```python
from build123d import *

# Parameters (mm, degrees)
EXTRUDE_1_DEPTH          = 2.5
SKETCH_4_R               = 1.6
CUT_EXTRUDE_1_DEPTH      = 2.5
SKETCH_6_R               = 29
SKETCH_6_R_2             = 27.5
EXTRUDE_2_DEPTH          = 20
CUT_EXTRUDE_2_DEPTH      = 86.473878076
CUT_EXTRUDE_2_DEPTH_BACK = 86.473878076
SKETCH_7_W               = 18
SKETCH_7_H               = 8


with BuildPart() as part:
    # 草图2 → 凸台-拉伸1 (new body)
    with BuildSketch(Plane(origin=(0, 0, 0), x_dir=(1, 0, 0), z_dir=(0, 1, 0))):
        Polygon((-42.5, 21.336828309), (42.5, 21.336828309), (42.5, -70.663171691), (32.5, -70.663171691), (-32.5, -70.663171691), (-42.5, -70.663171691), align=None)
    extrude(amount=EXTRUDE_1_DEPTH)

    # 草图4 → 切除-拉伸1 (cut)
    with BuildSketch(Plane(origin=(0, 2.5, 0), x_dir=(1, 0, 0), z_dir=(0, 1, 0))):
        with Locations(Location((-38.5, 18.393628901, 0), (0, 0, 270))):
            Circle(SKETCH_4_R)
        with Locations(Location((35.3, 18.393628901, 0), (0, 0, 270))):
            Circle(SKETCH_4_R)
        with Locations(Location((-31, -67.606371099, 0), (0, 0, 270))):
            Circle(SKETCH_4_R)
        with Locations(Location((27.8, -67.606371099, 0), (0, 0, 270))):
            Circle(SKETCH_4_R)
    extrude(amount=-CUT_EXTRUDE_1_DEPTH, mode=Mode.SUBTRACT)

    # 草图6 → 凸台-拉伸2 (add)
    with BuildSketch(Plane(origin=(0, 2.5, 0), x_dir=(1, 0, 0), z_dir=(0, 1, 0))):
        with Locations(Location((0, -24.663171691, 0), (0, 0, 270))):
            Circle(SKETCH_6_R)
        with Locations(Location((0, -24.663171691, 0), (0, 0, 270))):
            Circle(SKETCH_6_R_2, mode=Mode.SUBTRACT)
    extrude(amount=EXTRUDE_2_DEPTH)

    # 草图7 → 切除-拉伸2 (cut, two sides: drawn at the far end of the back side and taken through both)
    with BuildSketch(Plane(origin=(0, 0, 0), x_dir=(0, 0, -1), z_dir=(1, 0, 0)).offset(-CUT_EXTRUDE_2_DEPTH_BACK)):
        with Locations((-24.663171691, 6.5)):
            Rectangle(SKETCH_7_W, SKETCH_7_H)
    extrude(amount=CUT_EXTRUDE_2_DEPTH + CUT_EXTRUDE_2_DEPTH_BACK, mode=Mode.SUBTRACT)


solid = part.part
```
Verification items for the finished model (mm, model axes). A direction names the side the tool comes from. Round coordinates to 2 decimals unless told otherwise and drop trailing zeros. Write each loop counter-clockwise with the first axis right and the second up, starting at its lowest first coordinate (ties: lowest second). Pieces come first, ordered by that corner, then holes.
1. Draft check along Y on faces 4 (the flat face through (-28, 10.5, 25)), 5 (the cylindrical face through (-30.519, 1.268, 69.132)), 6 (the flat face through (22, 22.5, 42)). Enter one of: +Y half, -Y half, draft (parallel to the pull), parting line (faces both ways), or undercut.
2. Section check A-A on x = -31. Enter the section's corners in (y, z).
3. Access from +Z, -Z, +X, -X, +Y, -Y to the whole of each face (thin tool, end or side, straight path). Record for faces 1 (the cylindrical face through (-11.11, 12.36, 51.45)), 2 (the flat face through (28, 10.5, 25)), 3 (the flat face through (42.5, 1, 24)).
4. Scan lines: L1, parallel to Y at x = -17, z = 61; L2, parallel to X at y = 20, z = 15; L3, parallel to X at y = 15.5, z = 46. Record each from-to range of solid material in increasing order.
5. Section check B-B on x = 0. Enter the section's corners in (y, z).
6. Section check D-D on z = -5.5. Enter the section's corners in (x, y), plus the area to 4 significant figures.
7. Gauge pin test, flat ends, axial feed: P1, Ø2.5, axis at x = -31, z = 67.61, coming from the -Y side; P2, Ø1.7, axis at x = -27, y = 7, coming from the -Z side; P3, Ø0.5, axis at x = 26.5, y = 7.5, coming from the -Z side; P4, Ø8, axis at x = -11.5, y = 10, coming from the +Z side. Record the tip position at first contact, or that the pin passes through.
8. Section check C-C on z = 5.5. Enter the section's corners in (x, y), plus the area to 3 significant figures.
Answer:
1. face 4: undercut
1. face 5: draft
1. face 6: +Y half
2. outline: (0, -21.34) - (2.5, -21.34) - (2.5, 66.01) - (0, 66.01) - close; (0, 69.21) - (2.5, 69.21) - (2.5, 70.66) - (0, 70.66) - close
3. face 1: +Y
3. face 2: +X, -X
3. face 3: +Z, -Z, +X, +Y, -Y
4. L1: y = 0 to 2.5
4. L2: x = -27.34 to -25.75, 25.75 to 27.34
4. L3: x = -19.64 to -17.35, 17.35 to 19.64
5. outline: (0, -21.34) - (2.5, -21.34) - (2.5, -4.34) - (22.5, -4.34) - (22.5, -2.84) - (2.5, -2.84) - (2.5, 52.16) - (22.5, 52.16) - (22.5, 53.66) - (2.5, 53.66) - (2.5, 70.66) - (0, 70.66) - close
6. outline: (-42.5, 0) - (42.5, 0) - (42.5, 2.5) - (-42.5, 2.5) - close
6. area: 212.5 mm2
7. P1: passes through
7. P2: stops at z = 12.13
7. P3: stops at z = 12.34
7. P4: stops at z = 52.68
8. outline: (-42.5, 0) - (42.5, 0) - (42.5, 2.5) - (21.77, 2.5) - (21.77, 22.5) - (19.72, 22.5) - (19.72, 2.5) - (-19.72, 2.5) - (-19.72, 22.5) - (-21.77, 22.5) - (-21.77, 2.5) - (-42.5, 2.5) - close
8. area: 294 mm2
